from build123d import *

# Parameters (mm, degrees)
SKETCH1_R           = 20
BOSS_EXTRUDE1_DEPTH = 5
SKETCH2_R           = 15
CUT_EXTRUDE1_DEPTH  = 5
CUT_EXTRUDE2_START  = -5
CUT_EXTRUDE2_DEPTH  = 5
BOSS_EXTRUDE6_DEPTH = 5
BOSS_EXTRUDE7_DEPTH = 5
SKETCH13_R          = 1.5
CUT_EXTRUDE4_DEPTH  = 5
SKETCH14_R          = 1.5
BOSS_EXTRUDE8_DEPTH = 5


with BuildPart() as part:
    # Sketch1 → Boss-Extrude1 (new body)
    with BuildSketch(Plane(origin=(0, 0, 0), x_dir=(1, 0, 0), z_dir=(0, 1, 0))):
        with Locations(Location((0, 0, 0), (0, 0, 270))):
            Circle(SKETCH1_R)
    extrude(amount=BOSS_EXTRUDE1_DEPTH)

    # Sketch2 → Cut-Extrude1 (cut)
    with BuildSketch(Plane(origin=(0, 5, 0), x_dir=(1, 0, 0), z_dir=(0, 1, 0))):
        with Locations(Location((0, 0, 0), (0, 0, 270))):
            Circle(SKETCH2_R)
    extrude(amount=-CUT_EXTRUDE1_DEPTH, mode=Mode.SUBTRACT)

    # Sketch3 → Cut-Extrude2 (cut)
    with BuildSketch(Plane(origin=(0, 5, 0), x_dir=(1, 0, 0), z_dir=(0, 1, 0)).offset(CUT_EXTRUDE2_START)):
        with BuildLine():
            Line((6.840402867, 18.793852416), (0, 0))
            Line((0, 0), (-20, 0))
            ThreePointArc((-20, 0), (11.471528727, -16.383040886), (6.840402867, 18.793852416))
        make_face()
    extrude(amount=CUT_EXTRUDE2_DEPTH, mode=Mode.SUBTRACT)

    # Sketch10 → Boss-Extrude6 (add)
    with BuildSketch(Plane(origin=(0, 5, 0), x_dir=(1, 0, 0), z_dir=(0, 1, 0))):
        Polygon((5.13030215, 14.095389312), (81.360388775, -10.730274846), (82.988726433, -5.730274846), (6.840402867, 18.793852416), align=None)
    extrude(amount=-BOSS_EXTRUDE6_DEPTH)

    # Sketch12 → Boss-Extrude7 (add)
    with BuildSketch(Plane(origin=(0, 5, 0), x_dir=(1, 0, 0), z_dir=(0, 1, 0))):
        with BuildLine():
            Line((-20, 0), (-15, 0))
            ThreePointArc((-15, 0), (-17.5, -2.5), (-20, 0))
        make_face()
    extrude(amount=-BOSS_EXTRUDE7_DEPTH)

    # Sketch13 → Cut-Extrude4 (cut)
    with BuildSketch(Plane(origin=(0, 5, 0), x_dir=(1, 0, 0), z_dir=(0, 1, 0))):
        with Locations(Location((-17.5, 0, 0), (0, 0, 270))):
            Circle(SKETCH13_R)
    extrude(amount=-CUT_EXTRUDE4_DEPTH, mode=Mode.SUBTRACT)

    # Sketch14 → Boss-Extrude8 (add)
    with BuildSketch(Plane(origin=(0, 5, 0), x_dir=(1, 0, 0), z_dir=(0, 1, 0))):
        with Locations(Location((6.065841992, 16.416852345, 0), (0, 0, 270))):
            Circle(SKETCH14_R)
    extrude(amount=BOSS_EXTRUDE8_DEPTH)


solid = part.part
Model file for the job. Use its own axes, mm. A direction names the side the tool comes from. Round coordinates to 2 decimals unless told otherwise and drop trailing zeros. Loops run counter-clockwise (first coordinate to the right, second up) from the corner with the lowest first, then second, coordinate; pieces in that order, holes last. Notation, with made-up numbers: (23.5, 59) -> (76.5, 59) arc R26 ccw to (76.5, 82) -> close; hole circle Ø7 at (-22, 45). An arc over 180 degrees is marked (long way). Answer as CSV lines item,"result". Start each with the question number.
1) Slice it at C-C (x = -17.5). List the corners of the cut face in (y, z), plus the area to 3 significant figures.
2) Mould opens along Z. For faces 3 (the face through (-16.235, 2.535, 0.806)), 4 (the face through (32, 0, -6)), 5 (the face through (42.712, 2.535, -1.856)) say: +Z half, -Z half, draft (parallel to the pull), parting line (faces both ways), or undercut.
3) Slice it at A-A (y = 3.5). List the corners of the cut face in (x, z).
4) Tool access for faces 1 (the face through (6.516, 7.465, -14.986)), 2 (the face through (82.16, 2.54, 8.27)): list every direction of +Z, -Z, +X, -X, +Y, -Y with a clear straight run to the whole face (end or side of a thin tool).
5) Probe line 1 along Y through (x, z) = (71, 3); line 2 along Z through (x, y) = (44.5, 4.5); line 3 along Z through (x, y) = (27.5, 2.5). List the from-to ranges inside material, lowest first.
6) Slice it at D-D (z = 8). List the corners of the cut face in (x, y), plus the area to 3 significant figures.
7) Pin check, flat tips, straight feed: P1, Ø6, axis at y = 7.5, z = -8.5, coming from the -X side; P2, Ø6, axis at x = 4.5, y = 1, coming from the +Z side; P3, Ø6, axis at y = 6.5, z = -12.5, coming from the -X side. Stop position of each tip, or through.
8) Slice it at B-B (z = -3). List the corners of the cut face in (x, y), plus the area to 3 significant figures.
Filled in:
1,outline,"(0, -9.68) -> (5, -9.68) -> (5, -1.5) -> (0, -1.5) -> close; (0, 1.5) -> (5, 1.5) -> (5, 2.5) -> (0, 2.5) -> close"
1,area,"45.9 mm2"
2,face 3,"undercut"
2,face 4,"draft"
2,face 5,"+Z half"
3,outline,"(-20, 0) arc R20 ccw to (6.84, -18.79) -> (82.99, 5.73) -> (81.36, 10.73) -> (5.13, -14.1) arc R15 cw to (-15, 0) arc R2.5 ccw to start; hole circle Ø3 at (-17.5, 0)"
4,face 1,"+Y"
4,face 2,"+Z, +X, +Y, -Y"
5,line 1,"y = 0 to 5"
5,line 2,"z = -6.67 to -1.27"
5,line 3,"z = -12.14 to -6.81"
6,outline,"(72.98, 0) -> (82.25, 0) -> (82.25, 5) -> (72.98, 5) -> close"
6,area,"46.4 mm2"
7,P1,"stops at x = -18.79"
7,P2,"stops at z = -13.32"
7,P3,"stops at x = -17.38"
8,outline,"(-19.77, 0) -> (-14.7, 0) -> (-14.7, 5) -> (-19.77, 5) -> close; (39.2, 0) -> (55.88, 0) -> (55.88, 5) -> (39.2, 5) -> close"
8,area,"109 mm2"
